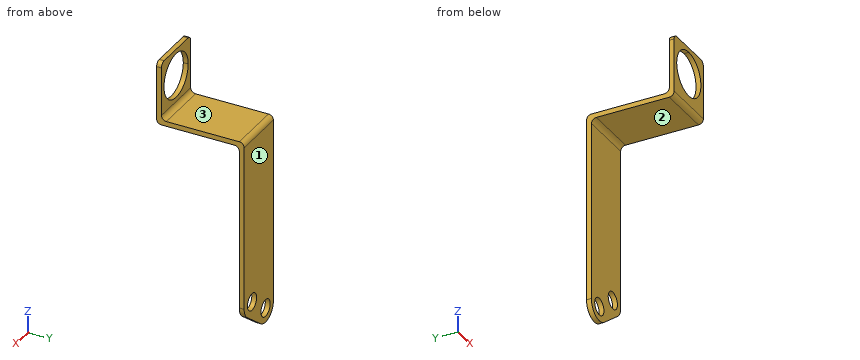
from build123d import *

# Parameters (mm, degrees)
F0_R     = 11.1125
F1_DEPTH = 6.35
F3_DEPTH = 70.7186416791
F5_DEPTH = 6.35
F7_DEPTH = 6.35


with BuildPart() as f1:
    # F0 (on Front) → F1 (new body)
    with BuildSketch(Plane.XZ):
        with BuildLine():
            Line((-174.6695893067, 281.6027870952), (-174.6695893067, 168.4105260595))
            ThreePointArc((-174.6695893067, 168.4105260595), (-164.4736790686, 150.5488967565), (-143.9870209187, 152.3630700653))
            Line((-143.9870209187, 152.3630700653), (-111.3431020089, 177.6217355725))
            ThreePointArc((-111.3431020089, 177.6217355725), (-105.8985434247, 184.2970768892), (-103.9509476276, 192.6881596848))
            Line((-103.9509476276, 192.6881596848), (-103.9509476276, 281.6027870952))
            Line((-103.9509476276, 281.6027870952), (-174.6695893067, 281.6027870952))
        make_face()
        with Locations((-155.6448665375, 167.4294941775)):
            Circle(F0_R, mode=Mode.SUBTRACT)
        with Locations((-123.0009476276, 192.6881596848)):
            Circle(F0_R, mode=Mode.SUBTRACT)
    extrude(amount=F1_DEPTH)

    # F2 (on face) → F3 (join, through all)
    with BuildSketch(Plane(origin=(-174.6695893067, 0, 0), x_dir=(0, -1, 0), z_dir=(-1, 0, 0))):
        with BuildLine():
            Line((0, 408.6027870952), (0, 281.6027870952))
            Line((0, 281.6027870952), (6.35, 281.6027870952))
            Line((6.35, 281.6027870952), (6.35, 402.2527870952))
            ThreePointArc((6.35, 402.2527870952), (8.2098719395, 406.7429151557), (12.7, 408.6027870952))
            Line((12.7, 408.6027870952), (107.95, 408.6027870952))
            ThreePointArc((107.95, 408.6027870952), (112.4401280605, 410.4626590346), (114.3, 414.9527870952))
            Line((114.3, 414.9527870952), (114.3, 491.1527870952))
            Line((114.3, 491.1527870952), (107.95, 491.1527870952))
            Line((107.95, 491.1527870952), (107.95, 421.3027870952))
            ThreePointArc((107.95, 421.3027870952), (106.0901280605, 416.8126590346), (101.6, 414.9527870952))
            Line((101.6, 414.9527870952), (6.35, 414.9527870952))
            ThreePointArc((6.35, 414.9527870952), (1.8598719395, 413.0929151557), (0, 408.6027870952))
        make_face()
    extrude(amount=-F3_DEPTH)

    # F4 (on face) → F5 (cut, through all)
    with BuildSketch(Plane(origin=(0, -107.95, 0), x_dir=(-1, 0, 0), z_dir=(0, 1, 0))):
        with BuildLine():
            ThreePointArc((139.3102684671, 485.4377870952), (118.6556793887, 435.5731980167), (168.5202684671, 456.2277870952))
            ThreePointArc((168.5202684671, 456.2277870952), (159.9648575456, 476.8823761736), (139.3102684671, 485.4377870952))
        make_face()
    extrude(amount=-F5_DEPTH, mode=Mode.SUBTRACT)

    # F6 (on face) → F7 (cut, through all)
    with BuildSketch(Plane(origin=(0, -107.95, 0), x_dir=(-1, 0, 0), z_dir=(0, 1, 0))):
        with BuildLine():
            ThreePointArc((103.9509476276, 484.8027870952), (105.8108195671, 489.2929151557), (110.3009476276, 491.1527870952))
            Line((110.3009476276, 491.1527870952), (103.9509476276, 491.1527870952))
            Line((103.9509476276, 491.1527870952), (103.9509476276, 484.8027870952))
        make_face()
        with BuildLine():
            Line((174.6695893067, 491.1527870952), (168.3195893067, 491.1527870952))
            ThreePointArc((168.3195893067, 491.1527870952), (172.8097173672, 489.2929151557), (174.6695893067, 484.8027870952))
            Line((174.6695893067, 484.8027870952), (174.6695893067, 491.1527870952))
        make_face()
    extrude(amount=-F7_DEPTH, mode=Mode.SUBTRACT)


solid = f1.part
Work out the finished part from the listing and answer in its coordinate system (mm). Face numbers are marked on the shaded views. A direction names the side the tool comes from. Round coordinates to 2 decimals unless told otherwise and drop trailing zeros. Write each loop counter-clockwise with the first axis right and the second up, starting at its lowest first coordinate (ties: lowest second). Pieces come first, ordered by that corner, then holes. Notation, with made-up numbers: (67, 80.25) - (102, 80.25) arc R22 ccw to (102, 103.25) - close; hole circle Ø7 at (19.25, 25.5). An arc over 180 degrees is marked (long way). Answer in a Markdown table with one row per item. Add a question column.
1. A cutting plane is placed at B-B, the plane y = -47.5. Determine the outline of the cut face in (x, z).
2. Given pin 1 (2 mm diameter, centred on x = -166, y = -65.5, fed in from -Z); pin 2 (8 mm diameter, centred on x = -167, y = -14, fed in from +Z); pin 3 (21 mm diameter, centred on x = -151, z = 459, fed in from +Y); pin 4 (4 mm diameter, centred on x = -142.5, z = 239.5, fed in from -Y), each flat-ended and moving along its own axis, determine where each tip first touches the part or whether it passes through.
3. For the marked faces 1, 2 and 3, determine the directions among +Z, -Z, +X, -X, +Y, -Y from which every point of the face is accessible in a straight line to the end or side of a thin tool.
4. A cutting plane is placed at C-C, the plane z = 380.5. Determine the outline of the cut face in (x, y), and give its area (3 significant figures).
5. A cutting plane is placed at A-A, the plane x = -151. Determine the outline of the cut face in (y, z).
6. Find the intervals of material crossed by line 1 along Y through (x, z) = (-167, 211); line 2 along X through (y, z) = (-74, 410); line 3 along Z through (x, y) = (-124, -91), in increasing order. Write a range as from..to.
7. A cutting plane is placed at D-D, the plane x = -122. Determine the outline of the cut face in (y, z).
Worked out:
| question | item | result |
|---|---|---|
| 1 | outline | (-174.67, 408.6) - (-103.95, 408.6) - (-103.95, 414.95) - (-174.67, 414.95) - close |
| 2 | pin 1 | z = 408.6 |
| 2 | pin 2 | z = 414.95 |
| 2 | pin 3 | through |
| 2 | pin 4 | y = -6.35 |
| 3 | face 1 | +Z, -Z, +X, -X, +Y |
| 3 | face 2 | -Z, +X, -X, -Y |
| 3 | face 3 | +Z, +X, -X, +Y |
| 4 | outline | (-174.67, -6.35) - (-103.95, -6.35) - (-103.95, 0) - (-174.67, 0) - close |
| 4 | area | 449 mm^2 |
| 5 | outline | (-114.3, 414.95) arc R6.35 ccw to (-107.95, 408.6) - (-12.7, 408.6) arc R6.35 cw to (-6.35, 402.25) - (-6.35, 177.52) - (0, 177.52) - (0, 408.6) arc R6.35 ccw to (-6.35, 414.95) - (-101.6, 414.95) arc R6.35 cw to (-107.95, 421.3) - (-107.95, 429.46) - (-114.3, 429.46) - close; (-114.3, 483) - (-107.95, 483) - (-107.95, 491.15) - (-114.3, 491.15) - close; (-6.35, 148.95) - (0, 148.95) - (0, 157.33) - (-6.35, 157.33) - close |
| 6 | line 1 | -6.35..0 |
| 6 | line 2 | -174.67..-103.95 |
| 6 | line 3 | 408.6..414.95 |
| 7 | outline | (-114.3, 414.95) arc R6.35 ccw to (-107.95, 408.6) - (-12.7, 408.6) arc R6.35 cw to (-6.35, 402.25) - (-6.35, 203.76) - (0, 203.76) - (0, 408.6) arc R6.35 ccw to (-6.35, 414.95) - (-101.6, 414.95) arc R6.35 cw to (-107.95, 421.3) - (-107.95, 432.7) - (-114.3, 432.7) - close; (-114.3, 479.76) - (-107.95, 479.76) - (-107.95, 491.15) - (-114.3, 491.15) - close; (-6.35, 169.38) - (0, 169.38) - (0, 181.62) - (-6.35, 181.62) - close |
